from build123d import *

# Parameters (mm, degrees)
PAD_DEPTH       = 25
POCKET_DEPTH    = 4
SKETCH002_R     = 2.5
POCKET001_DEPTH = 2.001


with BuildPart() as part:
    # Sketch → Pad (new body)
    with BuildSketch(Plane.YZ):
        Polygon((-5.25, -1.5), (5.25, -1.5), (5.25, 0), (8.75, 0), (6, 4.5), (-6, 4.5), (-8.75, 0), (-5.25, 0), align=None)
    extrude(amount=PAD_DEPTH)

    # Sketch001 (on Face5 of Pad) → Pocket (cut)
    with BuildSketch(Plane(origin=(0, 0, 4.5), x_dir=(0, -1, 0), z_dir=(0, 0, 1))):
        Polygon((4, 10.190599), (4, 14.809401), (0, 17.118802), (-4, 14.809401), (-4, 10.190599), (0, 7.881198), align=None)
    extrude(amount=-POCKET_DEPTH, mode=Mode.SUBTRACT)

    # Sketch002 (on Face17 of Pocket) → Pocket001 (cut, through all)
    with BuildSketch(Plane(origin=(0, 0, 0.5), x_dir=(0, -1, 0), z_dir=(0, 0, 1))):
        with Locations((0, 12.5)):
            Circle(SKETCH002_R)
    extrude(amount=-POCKET001_DEPTH, mode=Mode.SUBTRACT)


solid = part.part
The listing builds one solid part. Answer for the finished solid, in the listing's coordinates (mm). A direction names the side the tool comes from. Coordinates: 2 decimals unless noted, no trailing zeros. Write each loop counter-clockwise with the first axis right and the second up, starting at its lowest first coordinate (ties: lowest second). Pieces come first, ordered by that corner, then holes. Notation, with made-up numbers: (-24.5, 58) -> (30.5, 58) arc R16 cw to (30.5, 77) -> close; hole circle Ø5 at (12.25, 30.25). An arc over 180 degrees is marked (long way). One line per question, with ' | ' between items.
1. For a pull along X with two mould halves and no side action, classify faces 6 (the flat face through (25, 0, 2)), 7 (the flat face through (10, 4, 4.5)), 8 (the flat face through (13, 4, 3)) as released by +X, released by -X, zero draft, split by the parting line, or undercut.
Verdict:
face 6: released by +X | face 7: zero draft | face 8: undercut
2. Straight lines are drawn through the part: line 1 (X direction, y = 0, z = -0.5); line 2 (Y direction, x = 10, z = 3.5); line 3 (Y direction, x = 17.25, z = -0.75). For each, find the intervals that lie inside material, in ascending order.
Verdict:
line 1: x = 0 to 10, 15 to 25 | line 2: y = -6.61 to -3.67, 3.67 to 6.61 | line 3: y = -5.25 to 5.25
3. Section D-D (z = 1) is taken. Determine the outline of the cut face in (x, y).
Verdict:
outline: (0, -8.14) -> (25, -8.14) -> (25, 8.14) -> (0, 8.14) -> close; hole (7.88, 0) -> (10.19, -4) -> (14.81, -4) -> (17.12, 0) -> (14.81, 4) -> (10.19, 4) -> close
4. Section B-B (z = -0.75) is taken. Determine the outline of the cut face in (x, y).
Verdict:
outline: (0, -5.25) -> (25, -5.25) -> (25, 5.25) -> (0, 5.25) -> close; hole circle Ø5 at (12.5, 0)
5. Which of the six approach directions +Z, -Z, +X, -X, +Y, -Y give full straight-line access (tool end or side, diameter ignored) to faces 1 (the flat face through (12.325, -7.356, 2.281)), 2 (the flat face through (12, -4, 3)), 3 (the flat face through (12.325, 7.394, 2.219)), 4 (the flat face through (12, 7, 0)), 5 (the flat face through (12, -7, 0))?
Verdict:
face 1: +Z, +X, -X, -Y | face 2: +Z | face 3: +Z, +X, -X, +Y | face 4: -Z, +X, -X, +Y | face 5: -Z, +X, -X, -Y
6. Given pin 1 Ø1.5 at (x, z) = (22, 3) entering from -Y (3 decimals); pin 2 Ø0.8 at (x, z) = (7, -0.5) entering from +Y; pin 3 Ø1 at (x, y) = (9.5, -1) entering from +Z; pin 4 Ø3 at (x, y) = (12.5, 0) entering from +Z, each flat-ended and moving along its own axis, determine where each tip first touches the part or whether it passes through.
Verdict:
pin 1: stops at y = -7.375 | pin 2: stops at y = 5.25 | pin 3: stops at z = 0.5 | pin 4: passes through
7. Section C-C (x = 22) is taken. Determine the outline of the cut face in (y, z), and give its area (3 significant figures).
Verdict:
outline: (-8.75, 0) -> (-5.25, 0) -> (-5.25, -1.5) -> (5.25, -1.5) -> (5.25, 0) -> (8.75, 0) -> (6, 4.5) -> (-6, 4.5) -> close | area: 82.1 mm^2
8. Section A-A (x = 12.5) is taken. Determine the outline of the cut face in (y, z), and give its area (3 significant figures).
Verdict:
outline: (-8.75, 0) -> (-5.25, 0) -> (-5.25, -1.5) -> (-2.5, -1.5) -> (-2.5, 0.5) -> (-4, 0.5) -> (-4, 4.5) -> (-6, 4.5) -> close; (2.5, -1.5) -> (5.25, -1.5) -> (5.25, 0) -> (8.75, 0) -> (6, 4.5) -> (4, 4.5) -> (4, 0.5) -> (2.5, 0.5) -> close | area: 40.1 mm^2
